Build history of the part. All positions in model axes, mm. Give positions to 0.01 mm unless a question says otherwise; leave off trailing zeros. Write each loop counter-clockwise with the first axis right and the second up, starting at its lowest first coordinate (ties: lowest second). Pieces come first, ordered by that corner, then holes.
Autodesk Inventor part; units mm, degrees
ref_plane "YZ Plane" through (0, 0, 0) normal (1, 0, 0) x (0, 1, 0)
ref_plane "XZ Plane" through (0, 0, 0) normal (0, 1, 0) x (-1, 0, 0)
ref_plane "XY Plane" through (0, 0, 0) normal (0, 0, 1) x (1, 0, 0)
sketch "Sketch1" plane through (0, 0, 0) normal (0, 0, 1) x (1, 0, 0)
  circle A0 centre (-98.962, -47.4274) radius 2.1844
  circle A1 centre (39.6847, -45.4579) radius 2.9019 construction
  arc A2 (-100.8156, -41.354) -> (-98.7235, -53.773) centre (-98.962, -47.4274) ccw
  arc A3 (22.8757, -79.6496) -> (36.1943, -7.5182) centre (39.6847, -45.4579) ccw
  circle A4 centre (-11.8745, -21.7378) radius 6.35 construction
  arc A5 (-0.585, -10.9018) -> (-1.8569, -11.1517) centre (-0.0033, -17.2251) ccw
  line L0 (-11.8745, -21.7378) -> (-0.0033, -17.2251) construction
  line L1 (-98.962, -47.4274) -> (39.6847, -45.4579) construction
  circle A6 centre (-0.0033, -17.2251) radius 2.1844
  circle A7 centre (-11.8745, -21.7378) radius 2.1844
  line L2 (-100.8156, -41.354) -> (-1.8569, -11.1517)
  line L3 (36.1943, -7.5182) -> (-0.585, -10.9018)
  arc A8 (22.8757, -79.6496) -> (-98.7235, -53.773) centre (-89.1842, -307.5938) ccw
  circle A9 centre (39.6847, -45.4579) radius 4
  point P0 (0, 0)
  dimension "d0" = 12.7
  dimension "d1" = 76.2
  dimension "d2" = 12.7
  dimension "d3" = 20
  dimension "d4" = 4.3688
  dimension "d5" = 4.3688
  dimension "d6" = 254
  dimension "d7" = 8
extrude "Extrusion1" add sketch "Sketch1" along normal blind 5.08
properties part number "intakeside" material "Acetal Resin, Black"
1. Saw through at B-B on x = -80.5. Give the cut face in (y, z).
2. Saw through at C-C on y = -28. Give the cut face in (x, z), plus the area to 4 significant figures.
3. Saw through at A-A on z = 2.35. Give the cut face in (x, y) (1 decimal).
4. Drop flat-ended pins along their axis: pin 1 (2 mm diameter, centred on y = -56.5, z = 2, fed in from +X); pin 2 (3 mm diameter, centred on x = 13, z = 4.5, fed in from +Y); pin 3 (1.5 mm diameter, centred on x = -73.5, z = 3, fed in from +Y). Give the stop position or say it passes through.
5. Mould opens along X. For faces 1 (the face through (5, -45, 0)), 2 (the face through (-96.944, -46.591, 2.504)), 3 (the face through (77.318, -51.406, 2.504)) say: pulls with the +X half, pulls with the -X half, needs draft (parallel to the pull), parting line crosses it, or undercut.
6. Drill centre lines: line 1 along Y through (x, z) = (-44.5, 1.15); line 2 along Y through (x, z) = (-77, 1.95); line 3 along X through (y, z) = (-72, 3.85). Where is each one in solid material? Low to high.
Outcome:
1. outline: (-53.74, 0) - (-35.15, 0) - (-35.15, 5.08) - (-53.74, 5.08) - close
2. outline: (-57.06, 0) - (73.55, 0) - (73.55, 5.08) - (-57.06, 5.08) - close
2. area: 663.5 mm2
3. outline: (-100.8, -41.4) arc R6.4 ccw to (-98.7, -53.8) arc R254 cw to (22.9, -79.6) arc R38.1 ccw (long way) to (36.2, -7.5) - (-0.6, -10.9) arc R6.3 ccw to (-1.9, -11.2) - close; hole circle Ø4.4 at (-99, -47.4); hole circle Ø4.4 at (-11.9, -21.7); hole circle Ø4.4 at (0, -17.2); hole circle Ø8 at (39.7, -45.5)
4. pin 1: stops at x = 76.44
4. pin 2: stops at y = -9.51
4. pin 3: stops at y = -32.79
5. face 1: needs draft
5. face 2: undercut
5. face 3: parting line crosses it
6. line 1: y = -57.56 to -24.17
6. line 2: y = -53.89 to -34.09
6. line 3: x = 5.74 to 67.02
